Geometry: final body of the model. Coordinates: model frame, mm. Face numbers are marked on the shaded views. A direction names the side the tool comes from. Give positions to 0.01 mm unless a question says otherwise; leave off trailing zeros. Write each loop counter-clockwise with the first axis right and the second up, starting at its lowest first coordinate (ties: lowest second). Pieces come first, ordered by that corner, then holes. Notation, with made-up numbers: M 20,73 L 77,73 A31 ccw 77,112 Z; hole C 4,12 d9. An arc over 180 degrees is marked long. One line per question, with ' | ' between items.
from build123d import *

# Parameters (mm, degrees)
BASEHEAD_DEPTH     = 4.15
INDENT_START       = -0.51875
INDENT_2_OUTLINE_R = 4.375
INDENT_2_DEPTH     = 0.51875
SKETCH4_W          = 0.5
SKETCH4_H          = 10.773502692
THDSCHPAT_COUNT    = 18
THDSCHPAT_PITCH    = 1


# Read off the part's stored shape, not the designer's step: Indent
with BuildPart() as part:
    # Sketch1 → BaseHead (new body)
    with BuildSketch(Plane(origin=(0, 0, 0), x_dir=(0, 0, -1), z_dir=(1, 0, 0))):
        Polygon((5, 2.886751346), (5, -2.886751346), (0, -5.773502692), (-5, -2.886751346), (-5, 2.886751346), (0, 5.773502692), align=None)
    extrude(amount=BASEHEAD_DEPTH)

    # Indent outline → Indent (revolve)
    with BuildSketch(Plane.YX):
        Polygon((3, 4.15), (3, 38.5955), (2.4455, 39.15), (0, 39.15), (0, 4.15), align=None)
    revolve(axis=Axis((0, 0, 0), (1, 0, 0)))

    # Indent 2 outline → Indent 2 (cut)
    with BuildSketch(Plane.ZY.offset(INDENT_START)):
        with Locations((0.033212245, 0.192376607)):
            Circle(INDENT_2_OUTLINE_R)
    extrude(amount=INDENT_2_DEPTH, mode=Mode.SUBTRACT)

    # Sketch3 → HeadChamfer (revolve, cut)
    with BuildSketch(Plane.XY, mode=Mode.PRIVATE) as headchamfer_sk:
        Polygon((0, 5), (3.333333333, 10.773502692), (3.333333333, 15.773502692), (-10, 15.773502692), (-10, 5), align=None)
    revolve(headchamfer_sk.sketch.rotate(Axis((0, 0, 0), (1, 0, 0)), 90), axis=Axis((0, 0, 0), (1, 0, 0)), mode=Mode.SUBTRACT)

    # Sketch4 → BearingFace (revolve, cut)
    with BuildSketch(Plane.XY, mode=Mode.PRIVATE) as bearingface_sk:
        with Locations((3.9, 10.386751346)):
            Rectangle(SKETCH4_W, SKETCH4_H)
    revolve(bearingface_sk.sketch.rotate(Axis((0, 0, 0), (1, 0, 0)), 90), axis=Axis((0, 0, 0), (1, 0, 0)), mode=Mode.SUBTRACT)

    # ThdSchSke → ThreadSchematic (revolve, cut)
    with BuildSketch(Plane.XY):
        Polygon((21.15, -2.4455), (20.76173492, -3), (20.76173492, -3.75), (21.53826508, -3.75), (21.53826508, -3), align=None)
    threadschematic = revolve(axis=Axis((-3.175, 0, 0), (1, 0, 0)), mode=Mode.SUBTRACT)

    # ThdSchPat: ThreadSchematic ×18
    with Locations(*[(i * THDSCHPAT_PITCH, 0, 0) for i in range(1, THDSCHPAT_COUNT)]):
        add(threadschematic, mode=Mode.SUBTRACT)


solid = part.part
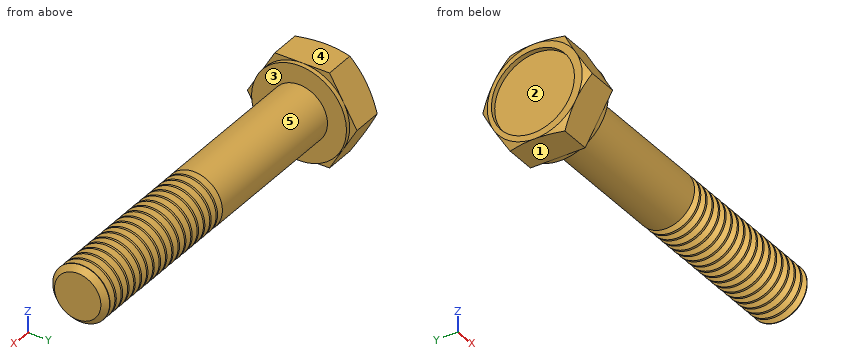
(1) Cut plane A-A, the plane x = 15. Return loops of the section in (y, z).
Working result:
outline: C 0,0 d6
(2) First-contact query: P1, Ø2.5, axis at y = -3, z = -3.5, coming from the +X side; P2, Ø6, axis at x = 26, y = 2, coming from the +Z side; P3, Ø3, axis at x = 9, y = -2.5, coming from the +Z side; P4, Ø3, axis at y = -4.5, z = -2, coming from the -X side. Flat tips, straight axial feed; report the tip coordinate or a pass-through.
Working result:
P1: stops at x = 4.15 | P2: stops at z = 3 | P3: stops at z = 2.83 | P4: stops at x = 0
(3) Draft query along Z for the marked faces 1, 2 and 3. Return one class per face: released by +Z, released by -Z, zero draft, split by the parting line, or undercut.
Working result:
face 1: released by -Z | face 2: undercut | face 3: zero draft
(4) Set-up query: the marked faces 4 and 5. Return all of +Z, -Z, +X, -X, +Y, -Y with unobstructed straight access to the full face (end or side cutting, diameter ignored); none if empty.
Working result:
face 4: +Z, +X, -X, +Y, -Y | face 5: +X
(5) Material intervals for L1, parallel to X at y = 0, z = 4.25; L2, parallel to X at y = -0.75, z = 4.75; L3, parallel to Z at x = 20, y = 2.75, sorted ascending. Write a range as [from, to].
Working result:
L1: x = [0.52, 4.15] | L2: x = [0, 4.15] | L3: z = [-1.2, 1.2]
